Read the model definition and answer for the solid it produces. Units are mm, in the model's axes. Face numbers are marked on the shaded views. Coordinates: 2 decimals unless noted, no trailing zeros. Write each loop counter-clockwise with the first axis right and the second up, starting at its lowest first coordinate (ties: lowest second). Pieces come first, ordered by that corner, then holes.
Item 1: Determine the mould class of the marked faces 1, 2, 3 and 4 for opening direction Z: released by +Z, released by -Z, zero draft, split by the parting line, or undercut.
Item 2: Section C-C (x = 24) is taken. Give the vertices of the cut face in (y, z).
Item 3: Straight lines are drawn through the part: probe 1 along Z at (x, y) = (-0.5, 22.75); probe 2 along X at (y, z) = (3.3, -21); probe 3 along Z at (x, y) = (-10.5, 20.5). For each, find the intervals that lie inside material, in ascending order.
Item 4: Each of these flat-tipped pins is pushed along its axis until it touches: P1, Ø5, axis at x = 23, y = 15, coming from the +Z side; P2, Ø6.5, axis at x = 0, z = -21, coming from the +Y side; P3, Ø5, axis at y = 15, z = -19.5, coming from the -X side; P4, Ø8, axis at y = 14, z = -7.5, coming from the -X side. Where does it stop, or does it pass through?
Item 5: Section A-A (z = 0) is taken. Give the vertices of the cut face in (x, y), then the cut area to 3 significant figures.
Item 6: Section B-B (z = -21) is taken. Give the vertices of the cut face in (x, y).
Item 7: Section D-D (y = 14) is taken. Give the vertices of the cut face in (x, z), then the cut area to 3 significant figures.
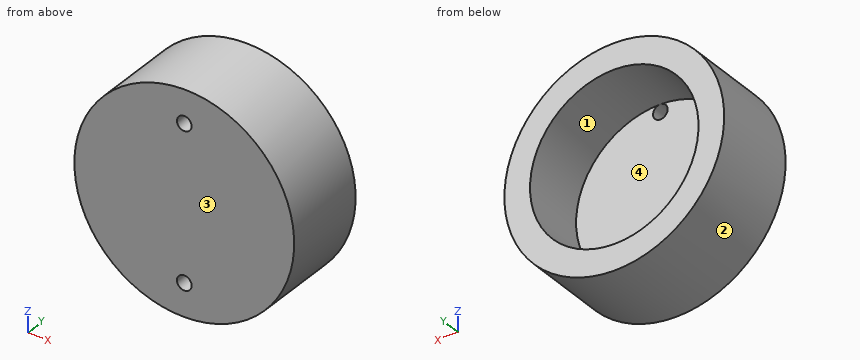
from build123d import *

# Parameters (mm, degrees)
SKETCH1_R           = 30
SKETCH1_R_2         = 23
BOSS_EXTRUDE1_DEPTH = 24
SKETCH1_2_R         = 23
BOSS_EXTRUDE2_DEPTH = 6
SKETCH2_R           = 2
CUT_EXTRUDE1_DEPTH  = 49.744230428


with BuildPart() as part:
    # Sketch1 → Boss-Extrude1 (new body)
    with BuildSketch(Plane(origin=(0, 0, 0), x_dir=(1, 0, 0), z_dir=(0, 1, 0))):
        with Locations(Location((0, 0, 0), (0, 0, 270))):
            Circle(SKETCH1_R)
        with Locations(Location((0, 0, 0), (0, 0, 270))):
            Circle(SKETCH1_R_2, mode=Mode.SUBTRACT)
    extrude(amount=BOSS_EXTRUDE1_DEPTH)

    # Sketch1_2 → Boss-Extrude2 (add)
    with BuildSketch(Plane(origin=(0, 0, 0), x_dir=(1, 0, 0), z_dir=(0, 1, 0))):
        with Locations(Location((0, 0, 0), (0, 0, 270))):
            Circle(SKETCH1_2_R)
    extrude(amount=BOSS_EXTRUDE2_DEPTH)

    # Sketch2 → Cut-Extrude1 (cut, through all)
    with BuildSketch(Plane.XZ):
        with Locations(Location((0, 21, 0), (0, 0, 270))):
            Circle(SKETCH2_R)
        with Locations(Location((0, -21, 0), (0, 0, 270))):
            Circle(SKETCH2_R)
    extrude(amount=-CUT_EXTRUDE1_DEPTH, mode=Mode.SUBTRACT)


solid = part.part
Established:
1. face 1: undercut
1. face 2: split by the parting line
1. face 3: zero draft
1. face 4: undercut
2. outline: (0, -18) - (24, -18) - (24, 18) - (0, 18) - close
3. probe 1: z = -30 to -22.99, 22.99 to 30
3. probe 2: x = -21.42 to -2, 2 to 21.42
3. probe 3: z = -28.1 to -20.46, 20.46 to 28.1
4. P1: stops at z = 21.9
4. P2: stops at y = 24
4. P3: stops at x = -24.72
4. P4: stops at x = -29.8
5. outline: (-30, 0) - (30, 0) - (30, 24) - (23, 24) - (23, 6) - (-23, 6) - (-23, 24) - (-30, 24) - close
5. area: 612 mm2
6. outline: (-21.42, 0) - (-2, 0) - (-2, 6) - (-9.38, 6) - (-9.38, 24) - (-21.42, 24) - close; (2, 0) - (21.42, 0) - (21.42, 24) - (9.38, 24) - (9.38, 6) - (2, 6) - close
7. outline: circle Ø60 at (0, 0); hole circle Ø46 at (0, 0)
7. area: 1,170 mm2
